```python
from build123d import *

# Parameters (mm, degrees)
SKETCH_W        = 13.739303
SKETCH_H        = 7.240993
PAD_DEPTH       = 10
FILLET_R        = 1
SKETCH001_R     = 1.912834
POCKET_DEPTH    = 10.001
SKETCH002_R     = 1.188533
SKETCH002_R_2   = 1.377063
POCKET001_DEPTH = 10.001
SKETCH003_W     = 2.814273
SKETCH003_H     = 4.040293
PAD001_DEPTH    = 10
FILLET001_R     = 1
FILLET002_R     = 0.5


with BuildPart() as part:
    # Sketch → Pad (new body)
    with BuildSketch(Plane.XY):
        with Locations((9.376143, 5.56999)):
            Rectangle(SKETCH_W, SKETCH_H)
    extrude(amount=PAD_DEPTH)

    # Fillet
    fillet_edges = [part.edges().sort_by_distance(p)[0] for p in [
        (16.245794, 1.949493, 5),
    ]]
    fillet(fillet_edges, radius=FILLET_R)

    # Sketch001 → Pocket (cut, through all)
    with BuildSketch(Plane.XY.offset(10)):
        with Locations((8.105963, 5.301824)):
            Circle(SKETCH001_R)
    extrude(amount=-POCKET_DEPTH, mode=Mode.SUBTRACT)

    # Sketch002 → Pocket001 (cut, through all)
    with BuildSketch(Plane.XY.offset(10)):
        with Locations((12.974515, 6.821315)):
            Circle(SKETCH002_R)
        with Locations((11.517051, 3.596284)):
            Circle(SKETCH002_R_2)
    extrude(amount=-POCKET001_DEPTH, mode=Mode.SUBTRACT)

    # Sketch003 → Pad001 (new body)
    with BuildSketch(Plane.XY.offset(10)):
        with Locations((4.507165, 6.656808)):
            Rectangle(SKETCH003_W, SKETCH003_H)
    extrude(amount=PAD001_DEPTH)

    # Fillet001
    fillet001_edges = [part.edges().sort_by_distance(p)[0] for p in [
        (5.914301, 4.636662, 15),
    ]]
    fillet(fillet001_edges, radius=FILLET001_R)

    # Fillet002
    fillet002_edges = [part.edges().sort_by_distance(p)[0] for p in [
        (5.914301, 7.156809, 10),
        (5.621408, 4.929555, 10),
        (4.007165, 4.636662, 10),
    ]]
    fillet(fillet002_edges, radius=FILLET002_R)


solid = part.part
```
CAD build for the part. Positions are in the model's coordinates, mm. A direction names the side the tool comes from. Round coordinates to 2 decimals unless told otherwise and drop trailing zeros. Loops run counter-clockwise (first coordinate to the right, second up) from the corner with the lowest first, then second, coordinate; pieces in that order, holes last. Notation, with made-up numbers: M 75,-14.5 L 112,-14.5 A21 cw 112,15.5 Z; hole C 26.25,-2 d5. An arc over 180 degrees is marked long. Return JSON: item names as keys, results as strings. Group by question number.
(1) Tool access for faces 4 (the flat face through (3.1, 6, 15)), 5 (the cylindrical face through (5.61, 4.92, 15.29)), 6 (the flat face through (5, 8.677, 15)), 7 (the flat face through (4, 4.637, 15)): list every direction of +Z, -Z, +X, -X, +Y, -Y with a clear straight run to the whole face (end or side of a thin tool).
(2) Mould opens along X. For faces 1 (the cylindrical face through (13.613, 7.823, 5.07)), 2 (the flat face through (5.914, 7, 15)), 3 (the flat face through (9, 9.19, 5)) say: +X half, -X half, draft (parallel to the pull), parting line (faces both ways), or undercut.
(3) Wall check: probe 1 along X at (y, z) = (6.75, 5.25); probe 2 along Z at (x, y) = (3.5, 3.5); probe 3 along X at (y, z) = (4.25, 4.75). Give the ranges that are in metal, low to high. Write a range as [from, to].
(4) Saw through at C-C, the plane y = 6.5. List the corners of the cut face in (x, z).
(5) Drop flat-ended pins along their axis: P1, Ø3, axis at x = 11.52, y = 3.6, coming from the +Z side; P2, Ø2.5, axis at y = 7, z = 16.5, coming from the -X side; P3, Ø0.5, axis at x = 4.5, z = 16, coming from the -Y side. Give the stop position or say it passes through.
(6) Saw through at B-B, the plane z = 16.25. List the corners of the cut face in (x, y), and give its area (3 significant figures).
(7) Saw through at D-D, the plane z = 2.25. List the corners of the cut face in (x, y), and give its area (3 significant figures).
(8) Saw through at A-A, the plane x = 13.5. List the corners of the cut face in (y, z).
Answer list:
{
 "1": {"face 4": "+Z, -X, +Y, -Y", "face 5": "+Z, +X, -Y", "face 6": "+Z, +X, -X, +Y", "face 7": "+Z, +X, -X, -Y"},
 "2": {"face 1": "undercut", "face 2": "+X half", "face 3": "draft"},
 "3": {"probe 1": "[2.51, 6.86], [9.36, 11.79], [14.16, 16.25]", "probe 2": "[0, 10]", "probe 3": "[2.51, 6.51], [9.7, 10.31], [12.73, 16.25]"},
 "4": {"outline": "M 2.51,0 L 6.61,0 L 6.61,10 L 6.41,10 A0.5 cw 5.91,10.5 L 5.91,20 L 3.1,20 L 3.1,10 L 2.51,10 Z; M 9.6,0 L 11.83,0 L 11.83,10 L 9.6,10 Z; M 14.12,0 L 16.25,0 L 16.25,10 L 14.12,10 Z"},
 "5": {"P1": "z = 10", "P2": "x = 3.1", "P3": "y = 4.64"},
 "6": {"outline": "M 3.1,4.64 L 4.91,4.64 A1 ccw 5.91,5.64 L 5.91,8.68 L 3.1,8.68 Z", "area": "11.2 mm2"},
 "7": {"outline": "M 2.51,1.95 L 15.25,1.95 A1 ccw 16.25,2.95 L 16.25,9.19 L 2.51,9.19 Z; hole C 8.11,5.3 d3.83; hole C 11.52,3.6 d2.75; hole C 12.97,6.82 d2.38", "area": "77.4 mm2"},
 "8": {"outline": "M 1.95,0 L 5.76,0 L 5.76,10 L 1.95,10 Z; M 7.89,0 L 9.19,0 L 9.19,10 L 7.89,10 Z"}
}
